Input: part model. Units: mm. Frame: model coordinates. Coordinates: 2 decimals unless noted, no trailing zeros. Loops run counter-clockwise (first coordinate to the right, second up) from the corner with the lowest first, then second, coordinate; pieces in that order, holes last. Notation, with made-up numbers: (-19.75, 42.5) -> (12.25, 42.5) arc R27 ccw to (12.25, 63.5) -> close; hole circle Ø9 at (32.5, -34). An arc over 180 degrees is marked (long way). Put each result on its own line as item: value. Start each with the question number.
1) Cut plane D-D (z = -20.5). Return the cut outline in (x, y), plus the area to 3 significant figures.
2) Material intervals for L1, parallel to X at y = 2.2, z = 0; L2, parallel to Z at x = 0, y = 2.25; L3, parallel to X at y = 1.9, z = -39, sorted ascending.
3) Cut plane B-B (y = 3.75). Return the cut outline in (x, z).
4) Cut plane A-A (x = 0). Return the cut outline in (y, z), plus the area to 3 significant figures.
5) Cut plane C-C (x = -29). Return the cut outline in (y, z).
Autodesk Inventor part; units mm, degrees
ref_plane "YZ Plane" through (0, 0, 0) normal (1, 0, 0) x (0, 1, 0)
ref_plane "XZ Plane" through (0, 0, 0) normal (0, 1, 0) x (-1, 0, 0)
ref_plane "XY Plane" through (0, 0, 0) normal (0, 0, 1) x (1, 0, 0)
sketch "スケッチ1" plane through (0, 0, 0) normal (0, 1, 0) x (-1, 0, 0)
  line L0 (25, 0) -> (-25, 0)
  line L1 (-25, 0) -> (-25, -105)
  line L2 (-25, -105) -> (25, -105)
  line L3 (25, -105) -> (25, 0)
  circle A0 centre (0, 0) radius 25
  circle A1 centre (0, 0) radius 57 construction
  circle A2 centre (0, 0) radius 75 construction
  circle A3 centre (0, 0) radius 10
  dimension "d0" = 114
  dimension "d2" = 150
  dimension "d4" = 20
  dimension "d5" = 50
  dimension "d28" = 105
extrude "押し出し1" add sketch "スケッチ1" along normal blind 5 contours A0 L0 A3 | L0 A3 A0 | L3 L2 L1 A0
sketch "スケッチ4" plane through (0, 5, 0) normal (0, 1, 0) x (1, 0, 0)
  line L0 (-60, 105) -> (60, 105)
  line L1 (60, 105) -> (60, 55)
  line L2 (60, 55) -> (-60, 55)
  line L3 (-60, 55) -> (-60, 105)
  line L4 (25, 105) -> (-25, 105)
  point P0 (0, 0)
  point P1 (0, 105)
  dimension "d24" = 50
  dimension "d25" = 120
extrude "押し出し4" add sketch "スケッチ4" against normal up to surface (5 mm away)
properties part number "ギアプレート_ギアなし"
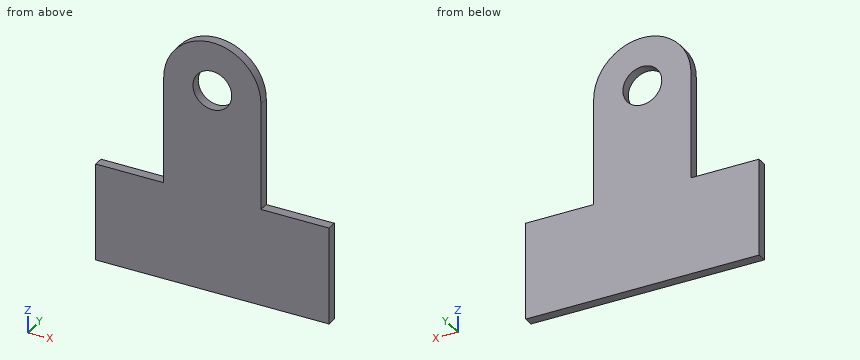
Results found:
1. outline: (-25, 0) -> (25, 0) -> (25, 5) -> (-25, 5) -> close
1. area: 250 mm2
2. L1: x = -25 to -10, 10 to 25
2. L2: z = -105 to -10, 10 to 25
2. L3: x = -25 to 25
3. outline: (-60, -105) -> (60, -105) -> (60, -55) -> (25, -55) -> (25, 0) arc R25 ccw to (-25, 0) -> (-25, -55) -> (-60, -55) -> close; hole circle Ø20 at (0, 0)
4. outline: (0, -105) -> (5, -105) -> (5, -10) -> (0, -10) -> close; (0, 10) -> (5, 10) -> (5, 25) -> (0, 25) -> close
4. area: 550 mm2
5. outline: (0, -105) -> (5, -105) -> (5, -55) -> (0, -55) -> close
